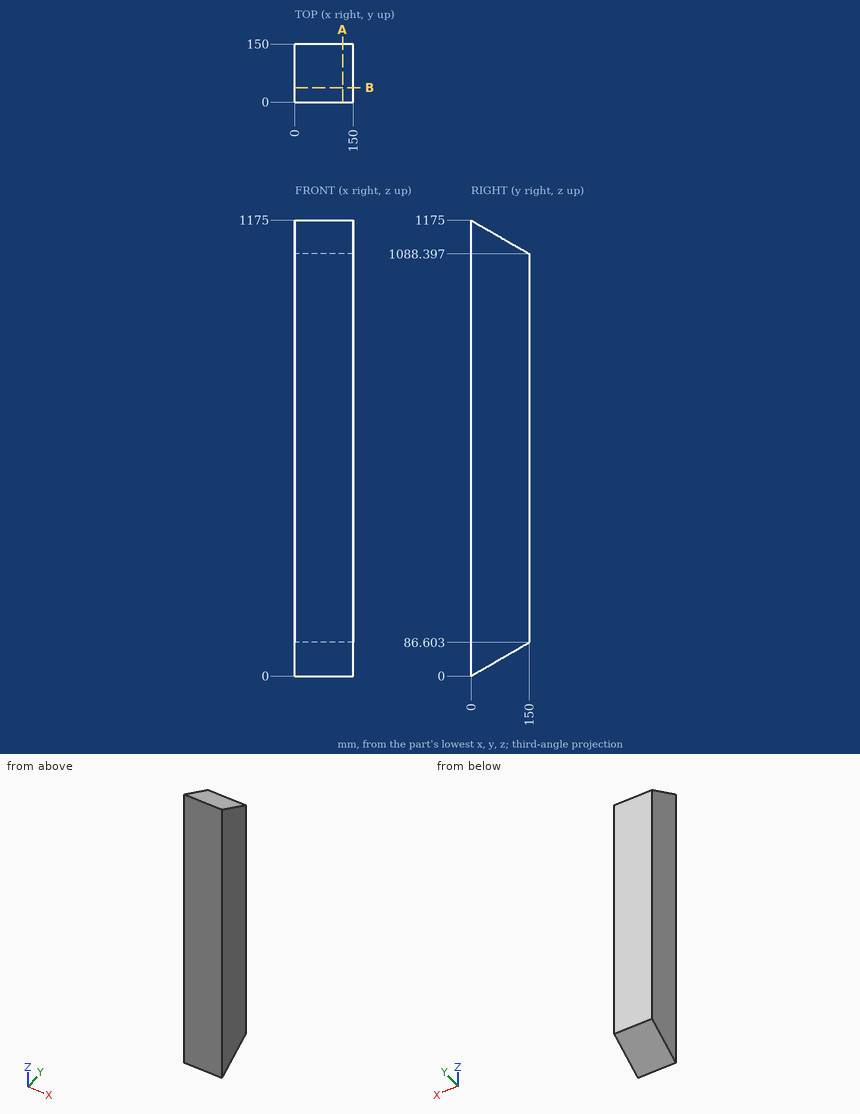
Source: three-view drawing plus pictorial views. Frame: mm from the lowest corner of the part. Give positions to 0.01 mm unless a question says otherwise; leave off trailing zeros. Order: outer loops, then holes, each group sorted by start corner. A loop starts at its lowest first (then second) coordinate and runs counter-clockwise, first axis right, second up. Notation, with made-up numbers: (44, -24) -> (97, -24) arc R7 cw to (97, -14) -> close; hole circle Ø5 at (39, -5.75). An arc over 180 degrees is marked (long way). Use a Markdown table: item, result.
Q1. Section A-A (x = 123). Return the cut outline in (y, z), and give its area (3 significant figures).
A:
| item | result |
|---|---|
| outline | (0, 0) -> (150, 86.6) -> (150, 1088.4) -> (0, 1175) -> close |
| area | 163,000 mm^2 |
Q2. Section B-B (y = 37.5). Return the cut outline in (x, z).
A:
| item | result |
|---|---|
| outline | (0, 21.65) -> (150, 21.65) -> (150, 1153.35) -> (0, 1153.35) -> close |
Q3. First-contact query: P1, Ø2, axis at x = 109, y = 53.5, coming from the -Z side; P2, Ø10, axis at x = 33, y = 106.5, coming from the +Z side; P3, Ø1, axis at y = 37.5, z = 342, coming from the -X side; P4, Ø1, axis at x = 43.5, y = 97.5, coming from the -Z side. Flat tips, straight axial feed; report the tip coordinate or a pass-through.
A:
| item | result |
|---|---|
| P1 | z = 30.31 |
| P2 | z = 1116.4 |
| P3 | x = 0 |
| P4 | z = 56 |
Q4. Material intervals for line 1 (Z direction, x = 50, y = 134) (1 decimal); line 2 (Z direction, x = 121, y = 88) (1 decimal), sorted ascending. Write a range as [from, to].
A:
| item | result |
|---|---|
| line 1 | [77.4, 1097.6] |
| line 2 | [50.8, 1124.2] |
